Can you work these out from the model? Positions are in its coordinate system, mm. Round coordinates to 2 decimals unless told otherwise and drop trailing zeros. Order: outer loops, then holes, each group sorted by start corner. A loop starts at its lowest first (then second) coordinate and runs counter-clockwise, first axis right, second up. Notation, with made-up numbers: (88.5, 38.25) -> (138.5, 38.25) arc R23 ccw to (138.5, 64.25) -> close; hole circle Ø10 at (19.5, 59). An arc over 180 degrees is marked (long way). One line per item, written item: value.
```python
from build123d import *

# Parameters (mm, degrees)
F0_W        = 15
F0_H        = 110
F1_DEPTH    = 105
F2_T1_DEPTH = 150


# Not quite as in the source:
# - a fillet or chamfer that OpenCascade refuses, or shapes differently, is made with other operations: its cross-section is extruded or revolved along the edge and cut away or added


with BuildPart() as f1:
    # F0 (on Top) → F1 (new body)
    with BuildSketch(Plane.XY):
        with Locations((1.6307681799, -0.1918845651)):
            Rectangle(F0_W, F0_H)
    extrude(amount=F1_DEPTH)

    # F2: fillet of radius 8 on 2 edges, made by hand

    # F2_s2 → F2_t1 (cut)
    with BuildSketch(Plane.XZ.offset(-74.8081154349)):
        with BuildLine():
            ThreePointArc((-5.8692318201, 97), (-3.5260860696, 102.6568542495), (2.1307681799, 105))
            Line((2.1307681799, 105), (-5.8692318201, 105))
            Line((-5.8692318201, 105), (-5.8692318201, 97))
        make_face()
        with BuildLine():
            ThreePointArc((9.1307681799, 97), (6.7876224294, 102.6568542495), (1.1307681799, 105))
            Line((1.1307681799, 105), (9.1307681799, 105))
            Line((9.1307681799, 105), (9.1307681799, 97))
        make_face()
    extrude(amount=F2_T1_DEPTH, mode=Mode.SUBTRACT)


solid = f1.part
```
Q1. I want a section at B-B on x = -3.25. List the corners of the cut face in (y, z) for me.
Answers below:
outline: (-55.19, 0) -> (54.81, 0) -> (54.81, 102.92) -> (-55.19, 102.92) -> close
Q2. I want a section at A-A on y = -30. List the corners of the cut face in (x, z) for me, plus the area to 3 significant figures.
Answers below:
outline: (-5.87, 0) -> (9.13, 0) -> (9.13, 97) arc R8 ccw to (1.63, 104.98) arc R8 ccw to (-5.87, 97) -> close
area: 1,550 mm^2
Q3. I want a section at C-C on x = 7.25. List the corners of the cut face in (y, z) for me, plus the area to 3 significant figures.
Answers below:
outline: (-55.19, 0) -> (54.81, 0) -> (54.81, 102.15) -> (-55.19, 102.15) -> close
area: 11,200 mm^2
Q4. Please list where these lines run through material, in increasing order: line 1 along Z through (x, y) = (-5, 41.5); line 2 along Z through (x, y) = (6.5, -13).
Answers below:
line 1: 0 to 100.63
line 2: 0 to 102.93
Q5. Will these pins go through, and if not, where does the flat tip stop? pin 1 Ø2 at (x, y) = (4, 43) entering from +Z; pin 2 Ø1 at (x, y) = (1, -17.5) entering from +Z.
Answers below:
pin 1: z = 104.78
pin 2: z = 104.98
